Job drawing, mm, ordinate dimensions from the low corner. One solid piece. Give positions to 0.01 mm unless a question says otherwise; leave off trailing zeros. Write each loop counter-clockwise with the first axis right and the second up, starting at its lowest first coordinate (ties: lowest second). Pieces come first, ordered by that corner, then holes. Notation, with made-up numbers: (62.5, 59.25) -> (85.5, 59.25) arc R31 cw to (85.5, 92.25) -> close; hole circle Ø11 at (75, -15.75). An arc over 180 degrees is marked (long way). Put each result on its own line as item: value. Start each with the question number.
Item 1: Slice it at A-A, the plane y = 0.5. Give the number of separate pieces and of enclosed holes in the cut face, plus the area to 3 significant figures.
Item 2: Flat gauge pins, fed straight in: pin 1 Ø1 at (y, z) = (1, 31.5) entering from -X; pin 2 Ø2 at (x, z) = (6.477, 2.921) entering from +Y; pin 3 Ø1 at (y, z) = (2, 16) entering from -X; pin 4 Ø1 at (x, y) = (7, 2) entering from +Z. Where does each tip first touch, or does it go through?
Item 3: Slice it at B-B, the plane z = 28. List the corners of the cut face in (x, y) (1 decimal).
Item 4: Drill centre lines: line 1 along Z through (x, y) = (89, 2) (1 decimal); line 2 along X through (y, z) = (1.75, 3); line 3 along X through (y, z) = (1.8, 23) (1 decimal). Where is each one in solid material? Low to high.
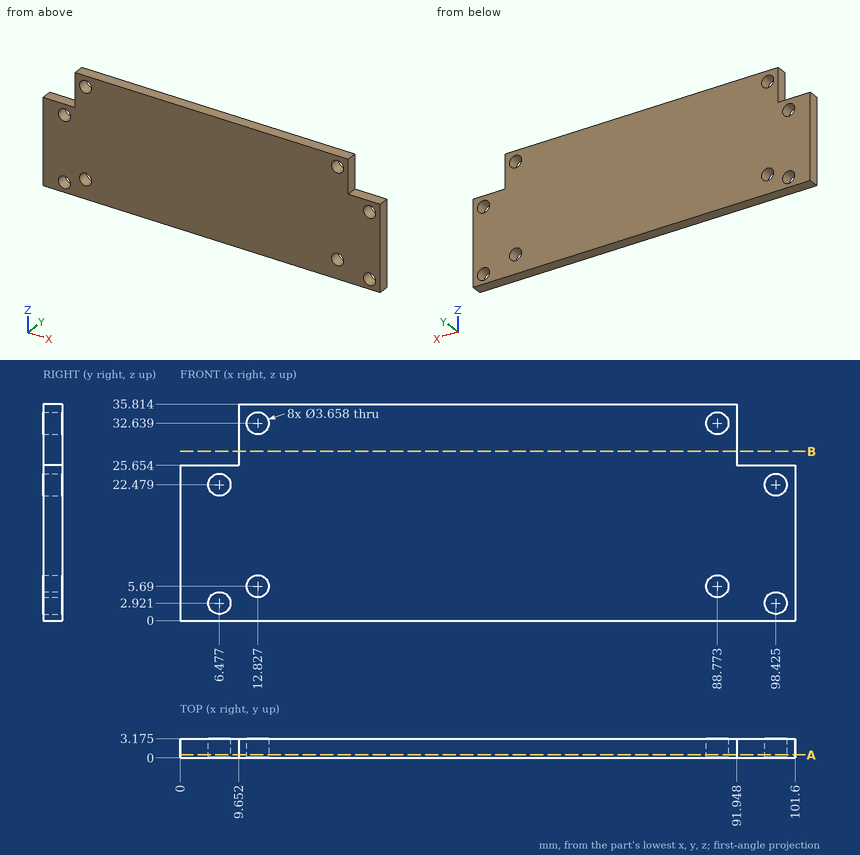
Values follow:
1. separate pieces: 1
1. enclosed holes: 8
1. area: 3,360 mm2
2. pin 1: x = 9.65
2. pin 2: through
2. pin 3: x = 0
2. pin 4: z = 25.65
3. outline: (9.7, 0) -> (91.9, 0) -> (91.9, 3.2) -> (9.7, 3.2) -> close
4. line 1: 0 to 3.9, 7.5 to 30.8, 34.5 to 35.8
4. line 2: 0 to 4.65, 8.3 to 96.6, 100.25 to 101.6
4. line 3: 0 to 4.7, 8.2 to 96.7, 100.2 to 101.6
